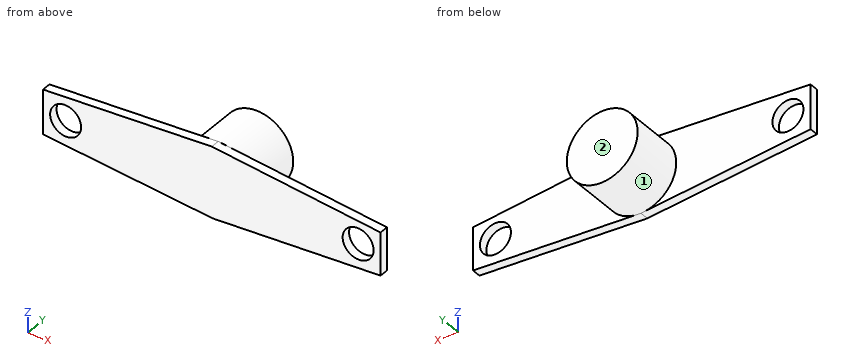
from build123d import *

# Parameters (mm, degrees)
CYLINDER023_R          = 1.75
CYLINDER023_DEPTH      = 17
CYLINDER023_ROLL_ANGLE = 90
CYLINDER022_R          = 1.75
CYLINDER022_DEPTH      = 17
CYLINDER022_ROLL_ANGLE = 90
PAD009_DEPTH           = 1
CYLINDER009_R          = 4
CYLINDER009_DEPTH      = 6
CYLINDER009_ROLL_ANGLE = 90


with BuildPart() as cylinder023:
    # Cylinder023 → Cylinder023 (new body)
    with BuildSketch(Plane.XY):
        Circle(CYLINDER023_R)
    extrude(amount=CYLINDER023_DEPTH)


with BuildPart() as cylinder023_1:
    # Cylinder023 roll: moved
    add(cylinder023.part.rotate(Axis((0, 0, 0), (1, 0, 0)), CYLINDER023_ROLL_ANGLE))


with BuildPart() as cylinder023_2:
    # Cylinder023 placement: moved
    add(cylinder023_1.part.moved(Location((-22, -12, 0))))


with BuildPart() as fusion002:
    # Cylinder022 → Cylinder022 (new body)
    with BuildSketch(Plane.XY):
        Circle(CYLINDER022_R)
    extrude(amount=CYLINDER022_DEPTH)


with BuildPart() as fusion002_1:
    # Cylinder022 roll: moved
    add(fusion002.part.rotate(Axis((0, 0, 0), (1, 0, 0)), CYLINDER022_ROLL_ANGLE))


with BuildPart() as fusion002_2:
    # Cylinder022 placement: moved
    add(fusion002_1.part.moved(Location((11, -12, 0))))

    # Fusion002: union Cylinder023
    add(cylinder023_2.part)


with BuildPart() as cut007:
    # Sketch008 → Pad009 (new body)
    with BuildSketch(Plane.XZ.offset(25)):
        Polygon((-24.552685, 2.449149), (-5.514274, 4), (13.531528, 2.326694), (13.531528, -2.510369), (-5.414014, -4), (-24.552685, -2.571598), align=None)
    extrude(amount=PAD009_DEPTH)

    # Cut007: cut Fusion002
    add(fusion002_2.part, mode=Mode.SUBTRACT)


with BuildPart() as fusion003:
    # Cylinder009 → Cylinder009 (new body)
    with BuildSketch(Plane.XY):
        Circle(CYLINDER009_R)
    extrude(amount=CYLINDER009_DEPTH)


with BuildPart() as fusion003_1:
    # Cylinder009 roll: moved
    add(fusion003.part.rotate(Axis((0, 0, 0), (1, 0, 0)), CYLINDER009_ROLL_ANGLE))


with BuildPart() as fusion003_2:
    # Cylinder009 placement: moved
    add(fusion003_1.part.moved(Location((-5.4, -19, 0))))

    # Fusion003: union Cut007
    add(cut007.part)


solid = fusion003_2.part
Check sheet for the modelled part. Datum: model origin and axes. Units: mm. Face numbers are marked on the shaded views. A direction names the side the tool comes from. Give positions to 0.01 mm unless a question says otherwise; leave off trailing zeros. Write each loop counter-clockwise with the first axis right and the second up, starting at its lowest first coordinate (ties: lowest second). Pieces come first, ordered by that corner, then holes. Notation, with made-up numbers: (40.25, 83) -> (63.25, 83) arc R4 ccw to (63.25, 89) -> close; hole circle Ø5 at (19, 37). An arc over 180 degrees is marked (long way). One line per item, written item: value. Start each with the question number.
Item 1: Tool access check on the marked faces 1 and 2. Record the directions out of +Z, -Z, +X, -X, +Y, -Y that give a thin tool (end or side, any length) a straight path to the whole face; none if there is none.
Item 2: Section check A-A on z = 0. Record the cut outline in (x, y).
Item 3: Section check D-D on x = -8. Record the cut outline in (y, z), then the cut area to 3 significant figures.
Item 4: Section check C-C on y = -22.5. Record the cut outline in (x, z).
Item 5: Gauge pin test, flat ends, axial feed: pin 1 (2.5 mm diameter, centred on x = -20, z = -1.5, fed in from +Y); pin 2 (3 mm diameter, centred on x = -2.5, y = -20, fed in from -Z); pin 3 (1.5 mm diameter, centred on x = -1, y = -22.5, fed in from +Z). Record the tip position at first contact, or that the pin passes through.
Item 6: Section check B-B on x = 10.5. Record the cut outline in (y, z), then the cut area to 3 significant figures.
Item 7: Material ranges on probe 1 along X at (y, z) = (-25.5, 1.5); probe 2 along Y at (x, z) = (-19, 1.25); probe 3 along Z at (x, y) = (11, -25.5), recorded low to high. Write a range as from..to.
Results list:
1. face 1: +Y
1. face 2: +Z, -Z, +X, -X, +Y
2. outline: (-24.55, -26) -> (-23.75, -26) -> (-23.75, -25) -> (-24.55, -25) -> close; (-20.25, -26) -> (9.25, -26) -> (9.25, -25) -> (-1.4, -25) -> (-1.4, -19) -> (-9.4, -19) -> (-9.4, -25) -> (-20.25, -25) -> close; (12.75, -26) -> (13.53, -26) -> (13.53, -25) -> (12.75, -25) -> close
3. outline: (-26, -3.81) -> (-25, -3.81) -> (-25, -3.04) -> (-19, -3.04) -> (-19, 3.04) -> (-25, 3.04) -> (-25, 3.8) -> (-26, 3.8) -> close
3. area: 44.1 mm²
4. outline: circle Ø8 at (-5.4, 0)
5. pin 1: y = -25
5. pin 2: z = -3.75
5. pin 3: z = 1.64
6. outline: (-26, -2.75) -> (-25, -2.75) -> (-25, -1.68) -> (-26, -1.68) -> close; (-26, 1.68) -> (-25, 1.68) -> (-25, 2.59) -> (-26, 2.59) -> close
6. area: 1.99 mm²
7. probe 1: -24.55..-22.9, -21.1..10.1, 11.9..13.53
7. probe 2: -26..-25
7. probe 3: -2.71..-1.75, 1.75..2.55
